from build123d import *

# Parameters (mm, degrees)
EXTRUDE_1_DEPTH     = 70
SKETCH_2_R          = 1.5
CUT_EXTRUDE_1_DEPTH = 10


with BuildPart() as part:
    # 草图1 → 凸台-拉伸1 (new body)
    with BuildSketch(Plane.XY):
        Polygon((0, 0), (30, 0), (30, 50), (170, 50), (170, 0), (200, 0), (200, -3), (167, -3), (167, 47), (33, 47), (33, -3), (0, -3), align=None)
    extrude(amount=EXTRUDE_1_DEPTH)

    # 草图2 → 切除-拉伸1 (cut)
    with BuildSketch(Plane(origin=(0, 50, 0), x_dir=(1, 0, 0), z_dir=(0, 1, 0))):
        with Locations(Location((123.018011593, -43.499999999, 0), (0, 0, 270))):
            Circle(SKETCH_2_R)
        with Locations(Location((136.441405352, -35.749999999, 0), (0, 0, 270))):
            Circle(SKETCH_2_R)
        with Locations(Location((136.441405352, -20.249999999, 0), (0, 0, 270))):
            Circle(SKETCH_2_R)
        with Locations(Location((123.018011593, -12.499999999, 0), (0, 0, 270))):
            Circle(SKETCH_2_R)
        with Locations(Location((109.594617835, -35.749999999, 0), (0, 0, 270))):
            Circle(SKETCH_2_R)
        with Locations(Location((109.594617835, -20.249999999, 0), (0, 0, 270))):
            Circle(SKETCH_2_R)
    extrude(amount=-CUT_EXTRUDE_1_DEPTH, mode=Mode.SUBTRACT)


solid = part.part
Geometry: final body of the model. Coordinates: model frame, mm. A direction names the side the tool comes from. Give positions to 0.01 mm unless a question says otherwise; leave off trailing zeros. Write each loop counter-clockwise with the first axis right and the second up, starting at its lowest first coordinate (ties: lowest second). Pieces come first, ordered by that corner, then holes. Notation, with made-up numbers: (51, 33) -> (93, 33) arc R30 ccw to (93, 55) -> close; hole circle Ø3 at (47, -30). An arc over 180 degrees is marked (long way). Answer in a Markdown table with one row per item.
(1) Draft query along X for faces 5 (the flat face through (167, 22, 35)), 6 (the flat face through (185, 0, 35)), 7 (the flat face through (30, 25, 35)). Return one class per face: +X half, -X half, draft (parallel to the pull), parting line (faces both ways), or undercut.
Answers below:
| item | result |
|---|---|
| face 5 | undercut |
| face 6 | draft |
| face 7 | -X half |
(2) Section query B-B on z = 65. Return loops of the section in (x, y).
Answers below:
| item | result |
|---|---|
| outline | (0, -3) -> (33, -3) -> (33, 47) -> (167, 47) -> (167, -3) -> (200, -3) -> (200, 0) -> (170, 0) -> (170, 50) -> (30, 50) -> (30, 0) -> (0, 0) -> close |
(3) Pin query (flat end, axial travel): pin 1 (2 mm diameter, centred on y = 34, z = 21.5, fed in from +X); pin 2 (5 mm diameter, centred on y = 6, z = 53.5, fed in from -X); pin 3 (2.5 mm diameter, centred on x = 109.59, z = 35.75, fed in from +Y); pin 4 (3.5 mm diameter, centred on x = 136.44, z = 20.25, fed in from +Y). Return the tip coordinate at first contact, or that it passes through.
Answers below:
| item | result |
|---|---|
| pin 1 | x = 170 |
| pin 2 | x = 30 |
| pin 3 | through |
| pin 4 | y = 50 |
(4) Set-up query: faces 1 (the flat face through (122.7, 47.2, 70)), 2 (the flat face through (170, 25, 35)), 3 (the flat face through (15, 0, 35)), 4 (the flat face through (101, 47, 35)). Return all of +Z, -Z, +X, -X, +Y, -Y with unobstructed straight access to the full face (end or side cutting, diameter ignored); none if empty.
Answers below:
| item | result |
|---|---|
| face 1 | +Z, +X, -X, +Y, -Y |
| face 2 | +Z, -Z, +X, +Y |
| face 3 | +Z, -Z, -X, +Y |
| face 4 | +Z, -Z, -Y |
(5) Section query A-A on y = 41.5. Return loops of the section in (x, z), then the cut area to 3 significant figures.
Answers below:
| item | result |
|---|---|
| outline | (30, 0) -> (33, 0) -> (33, 70) -> (30, 70) -> close; (167, 0) -> (170, 0) -> (170, 70) -> (167, 70) -> close |
| area | 420 mm^2 |
(6) Section query C-C on x = 164. Return loops of the section in (y, z).
Answers below:
| item | result |
|---|---|
| outline | (47, 0) -> (50, 0) -> (50, 70) -> (47, 70) -> close |
(7) Ray query, line 1 along X through (y, z) = (10.5, 16); line 2 along X through (y, z) = (47.7, 43.5); line 3 along Y through (x, z) = (77, 58). Return the intervals inside material, ascending. Write a range as [from, to].
Answers below:
| item | result |
|---|---|
| line 1 | [30, 33], [167, 170] |
| line 2 | [30, 121.52], [124.52, 170] |
| line 3 | [47, 50] |
